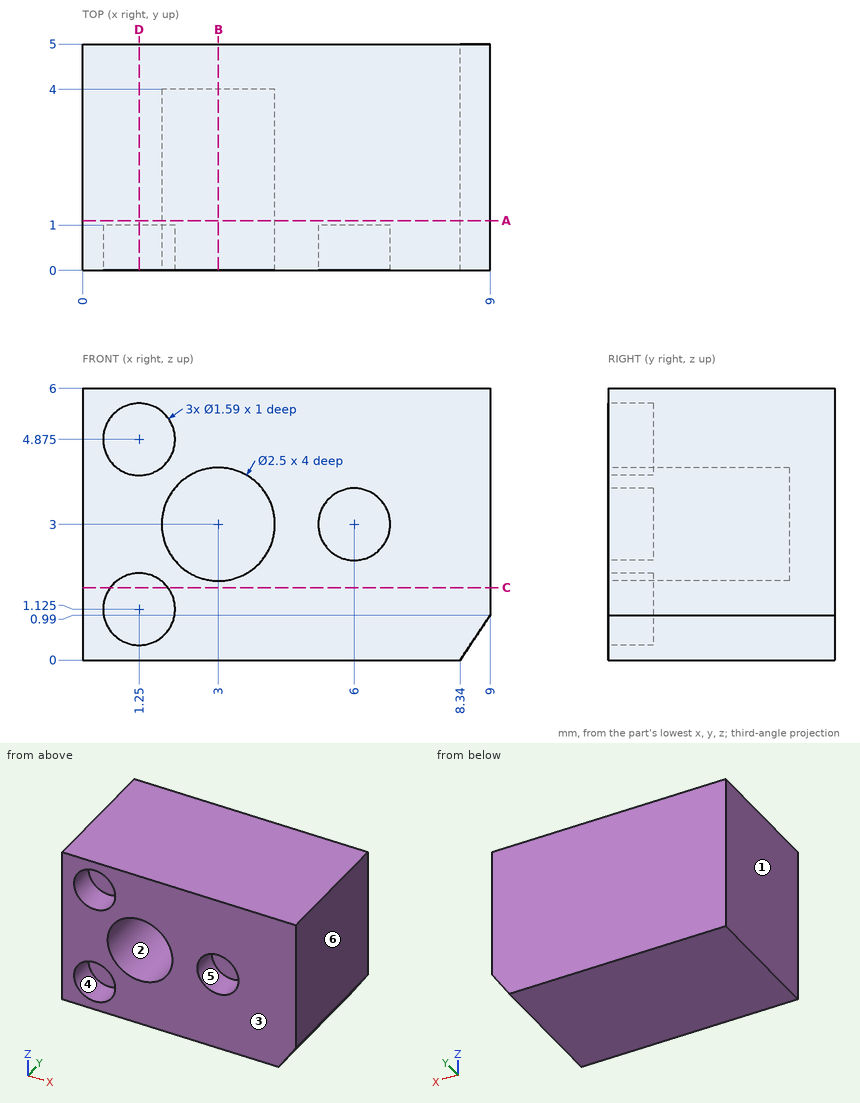
Input: dimensioned drawing with shaded views. Units: mm. Origin: part minimum x, y, z. A direction names the side the tool comes from. Give positions to 0.01 mm unless a question says otherwise; leave off trailing zeros. Loops run counter-clockwise (first coordinate to the right, second up) from the corner with the lowest first, then second, coordinate; pieces in that order, holes last. Notation, with made-up numbers: (29.5, -27.75) -> (36.5, -27.75) arc R23 cw to (36.5, 4.25) -> close; hole circle Ø5 at (51, 45). An arc over 180 degrees is marked (long way). Use a Markdown table: item, result. Add a question column.
1) Section query A-A, the plane y = 1.1. Return the cut outline in (x, z), then the cut area to 3 significant figures.
2) Section query D-D, the plane x = 1.25. Return the cut outline in (y, z).
3) Section query B-B, the plane x = 3. Return the cut outline in (y, z), then the cut area to 3 significant figures.
4) Pull-direction query (X, two-part tool) for the marked faces 1, 2, 3 and 4; classes: +X half, -X half, draft (parallel to the pull), parting line (faces both ways), or undercut.
5) Line query: line 1 along Z through (x, y) = (1.25, 0.4); line 2 along Z through (x, y) = (5.5, 0.4); line 3 along Y through (x, z) = (2.5, 3.8). Output: solid intervals per line, ascending. Write a range as [from, to].
6) First-contact query: pin 1 (0.8 mm diameter, centred on x = 1.5, z = 1, fed in from -Y). Flat tip, straight axial feed; report the tip coordinate or a pass-through.
7) Section query C-C, the plane z = 1.6. Return the cut outline in (x, y), then the cut area to 3 significant figures.
8) Reachability of the marked faces 5 and 6 from +Z, -Z, +X, -X, +Y, -Y: full face, straight path, thin tool, end or side. Return the list, or none.
Numbers:
| question | item | result |
|---|---|---|
| 1 | outline | (0, 0) -> (8.34, 0) -> (9, 0.99) -> (9, 6) -> (0, 6) -> close; hole circle Ø2.5 at (3, 3) |
| 1 | area | 48.8 mm2 |
| 2 | outline | (0, 0) -> (5, 0) -> (5, 6) -> (0, 6) -> (0, 5.67) -> (1, 5.67) -> (1, 4.08) -> (0, 4.08) -> (0, 1.92) -> (1, 1.92) -> (1, 0.33) -> (0, 0.33) -> close |
| 3 | outline | (0, 0) -> (5, 0) -> (5, 6) -> (0, 6) -> (0, 4.25) -> (4, 4.25) -> (4, 1.75) -> (0, 1.75) -> close |
| 3 | area | 20.0 mm2 |
| 4 | face 1 | -X half |
| 4 | face 2 | undercut |
| 4 | face 3 | draft |
| 4 | face 4 | undercut |
| 5 | line 1 | z = [0, 0.33], [1.92, 4.08], [5.67, 6] |
| 5 | line 2 | z = [0, 2.38], [3.62, 6] |
| 5 | line 3 | y = [4, 5] |
| 6 | pin 1 | stops at y = 1 |
| 7 | outline | (0, 0) -> (0.61, 0) -> (0.61, 1) -> (1.89, 1) -> (1.89, 0) -> (9, 0) -> (9, 5) -> (0, 5) -> close |
| 7 | area | 43.7 mm2 |
| 8 | face 5 | -Y |
| 8 | face 6 | +Z, -Z, +X, +Y, -Y |
